```python
from build123d import *

# Parameters (mm, degrees)
SKETCH1_W               = 455.168
SKETCH1_H               = 201.168
BOSS_EXTRUDE1_DEPTH     = 1.5875
F_1_4_CLEARANCE_HOLE1_D = 6.7564
CUT_EXTRUDE1_REACH      = 250.826
SKETCH4_R               = 17.4625
F_1_4_CLEARANCE_HOLE2_D = 6.7564
CUT_EXTRUDE2_REACH      = 250.826
SKETCH7_W               = 6.7564
SKETCH7_H               = 14.478
CHAMFER1_SIZE           = 6.35


with BuildPart() as part:
    # Sketch1 → Boss-Extrude1 (new body)
    with BuildSketch(Plane.XY):
        Rectangle(SKETCH1_W, SKETCH1_H)
    extrude(amount=BOSS_EXTRUDE1_DEPTH)

    # 1/4 Clearance Hole1 (through all)
    with Locations(Plane.XY.offset(1.5875)):
        with Locations((-203.2, 87.884), (203.2, 87.884), (-203.2, -87.884), (203.2, -87.884)):
            Hole(F_1_4_CLEARANCE_HOLE1_D / 2)

    # Sketch4 → Cut-Extrude1 (cut, up to next)
    with BuildSketch(Plane.XY.offset(1.5875), mode=Mode.PRIVATE) as cut_extrude1_sk1:
        with Locations((100.584, 0)):
            Circle(SKETCH4_R)
    cut_extrude1_tool1 = extrude(cut_extrude1_sk1.sketch, amount=-CUT_EXTRUDE1_REACH, mode=Mode.PRIVATE) & part.part
    add(cut_extrude1_tool1.solids().sort_by_distance((100.584, 0, 1.5875))[0], mode=Mode.SUBTRACT)

    # 1/4 Clearance Hole2 (through all)
    with Locations(Plane.XY.offset(1.5875)):
        with Locations((0, -87.884), (0, 87.884)):
            Hole(F_1_4_CLEARANCE_HOLE2_D / 2)

    # Sketch7 → Cut-Extrude2 (cut, up to next)
    with BuildSketch(Plane.XY.offset(1.5875), mode=Mode.PRIVATE) as cut_extrude2_sk1:
        with Locations((-203.2, -95.123)):
            Rectangle(SKETCH7_W, SKETCH7_H)
    cut_extrude2_tool1 = extrude(cut_extrude2_sk1.sketch, amount=-CUT_EXTRUDE2_REACH, mode=Mode.PRIVATE) & part.part
    # Sketch7 → Cut-Extrude2 (cut, up to next)
    with BuildSketch(Plane.XY.offset(1.5875), mode=Mode.PRIVATE) as cut_extrude2_sk2:
        with Locations((0, -95.123)):
            Rectangle(SKETCH7_W, SKETCH7_H)
    cut_extrude2_tool2 = extrude(cut_extrude2_sk2.sketch, amount=-CUT_EXTRUDE2_REACH, mode=Mode.PRIVATE) & part.part
    # Sketch7 → Cut-Extrude2 (cut, up to next)
    with BuildSketch(Plane.XY.offset(1.5875), mode=Mode.PRIVATE) as cut_extrude2_sk3:
        with Locations((203.2, -95.123)):
            Rectangle(SKETCH7_W, SKETCH7_H)
    cut_extrude2_tool3 = extrude(cut_extrude2_sk3.sketch, amount=-CUT_EXTRUDE2_REACH, mode=Mode.PRIVATE) & part.part
    cut_extrude2_1 = cut_extrude2_tool1.solids().sort_by_distance((-203.2, -95.123, 1.5875))[0]
    add(cut_extrude2_1, mode=Mode.SUBTRACT)
    cut_extrude2_2 = cut_extrude2_tool2.solids().sort_by_distance((0, -95.123, 1.5875))[0]
    add(cut_extrude2_2, mode=Mode.SUBTRACT)
    cut_extrude2_3 = cut_extrude2_tool3.solids().sort_by_distance((203.2, -95.123, 1.5875))[0]
    add(cut_extrude2_3, mode=Mode.SUBTRACT)
    cut_extrude2 = cut_extrude2_1 + cut_extrude2_2 + cut_extrude2_3  # Cut-Extrude2 as one shape, for the pattern or mirror that repeats it

    # Mirror1: Cut-Extrude2 across plane
    add(cut_extrude2.mirror(Plane.ZX), mode=Mode.SUBTRACT)

    # Chamfer1
    chamfer1_edges = [part.edges().sort_by_distance(p)[0] for p in [
        (227.584, -100.584, 0.79375),
        (-227.584, -100.584, 0.79375),
        (-227.584, 100.584, 0.79375),
        (227.584, 100.584, 0.79375),
    ]]
    chamfer(chamfer1_edges, length=CHAMFER1_SIZE)


solid = part.part
```
Here's how the part is built. I have some questions about the finished solid (model axes, mm). Give positions to 0.01 mm unless a question says otherwise; leave off trailing zeros. Loops run counter-clockwise (first coordinate to the right, second up) from the corner with the lowest first, then second, coordinate; pieces in that order, holes last. Notation, with made-up numbers: (50.5, 23.25) -> (81.5, 23.25) arc R25 ccw to (81.5, 36.25) -> close; hole circle Ø11 at (-21, 62). An arc over 180 degrees is marked (long way). Use one line per item in the form item = value. Start each with the question number.
1) Imagine slicing it at C-C (x = 99.5). Please give me the cut outline in (y, z), then the cut area to 3 significant figures.
2) For P1, Ø0.8, axis at y = 96, z = 1, coming from the +X side; P2, Ø0.8, axis at y = -97, z = 1, coming from the +X side; P3, Ø0.8, axis at y = 95, z = 1, coming from the +X side, each with a flat end and sliding along its axis, tell me the tip position at first contact or that it passes through.
3) Imagine slicing it at A-A (y = 0). Please give me the cut outline in (x, z), then the cut area to 3 significant figures.
4) Thinking about a two-plate mould opening in X: for faces 1 (the face through (-3, 1, 1.588)), 2 (the face through (117.24, 5.25, 0.8)), which applies, +X half, -X half, draft (parallel to the pull), parting line (faces both ways), or undercut?
Check values:
q1.outline = (-100.58, 0) -> (-17.43, 0) -> (-17.43, 1.59) -> (-100.58, 1.59) -> close; (17.43, 0) -> (100.58, 0) -> (100.58, 1.59) -> (17.43, 1.59) -> close
q1.area = 264 mm^2
q2.P1 = 226.22
q2.P2 = 225.22
q2.P3 = 227.22
q3.outline = (-227.58, 0) -> (83.12, 0) -> (83.12, 1.59) -> (-227.58, 1.59) -> close; (118.05, 0) -> (227.58, 0) -> (227.58, 1.59) -> (118.05, 1.59) -> close
q3.area = 667 mm^2
q4.face_1 = draft
q4.face_2 = undercut
